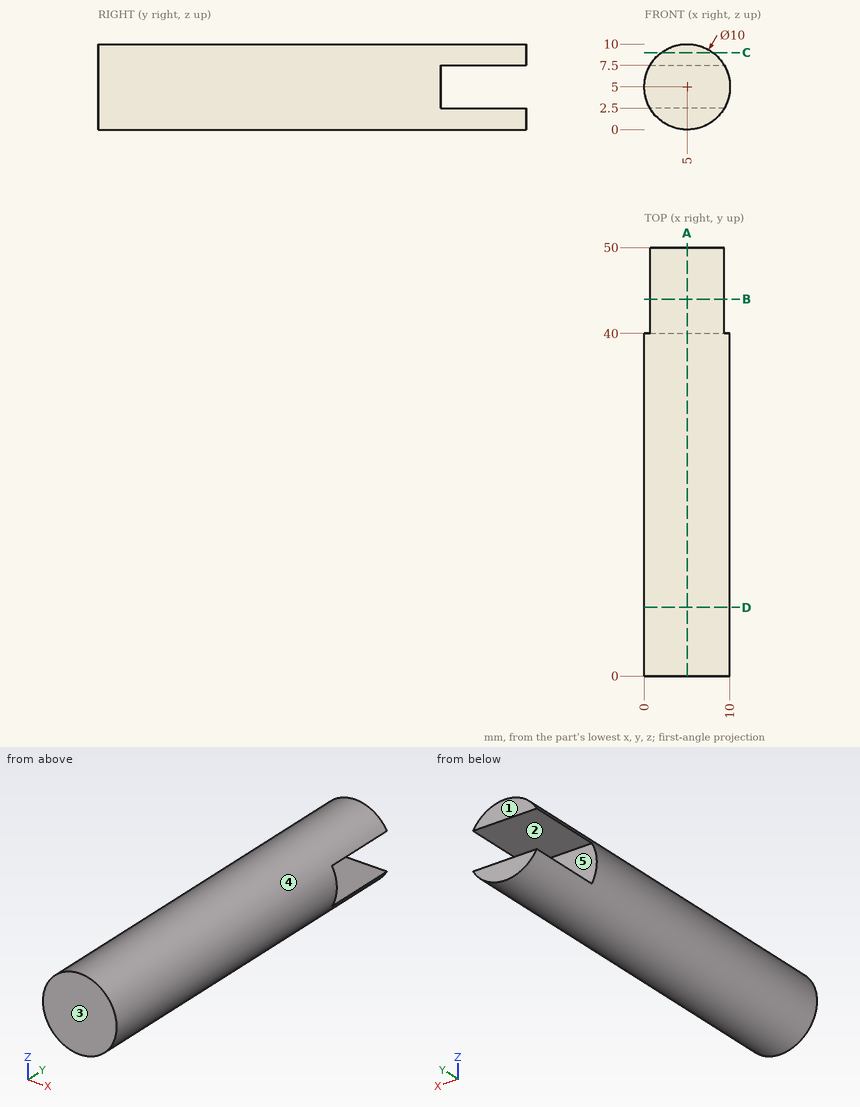
Source: three-view drawing plus pictorial views. Frame: mm from the lowest corner of the part. A direction names the side the tool comes from. Give positions to 0.01 mm unless a question says otherwise; leave off trailing zeros. Order: outer loops, then holes, each group sorted by start corner. A loop starts at its lowest first (then second) coordinate and runs counter-clockwise, first axis right, second up. Notation, with made-up numbers: M -34,-19 L -18,-19 A11 ccw -18,-4 Z; hole C 77.5,23.5 d5. An arc over 180 degrees is marked long. Return JSON: item names as keys, results as strings.
Item 1: First-contact query: P1, Ø1, axis at y = 38, z = 4, coming from the +X side; P2, Ø1.5, axis at x = 8, y = 44.5, coming from the -Z side; P3, Ø4, axis at x = 4, z = 4, coming from the +Y side; P4, Ø1, axis at y = 24, z = 8, coming from the -X side. Flat tips, straight axial feed; report the tip coordinate or a pass-through.
Solutions:
{"P1": "x = 9.97", "P2": "z = 0.53", "P3": "y = 50", "P4": "x = 0.67"}
Item 2: Cut plane C-C (z = 9). Return loops of the section in (x, y).
Solutions:
{"outline": "M 2,0 L 8,0 L 8,50 L 2,50 Z"}
Item 3: Cut plane B-B (y = 44). Return loops of the section in (x, z), then the cut area to 3 significant figures.
Solutions:
{"outline": "M 0.67,2.5 A5 ccw 9.33,2.5 Z; M 0.67,7.5 L 9.33,7.5 A5 ccw Z", "area": "30.7 mm^2"}
Item 4: Pull-direction query (Z, two-part tool) for the marked faces 3, 4 and 5; classes: +Z half, -Z half, draft (parallel to the pull), parting line (faces both ways), or undercut.
Solutions:
{"face 3": "draft", "face 4": "parting line", "face 5": "undercut"}
Item 5: Access query for the marked faces 1 and 2. Directions: +Z, -Z, +X, -X, +Y, -Y. A direction counts if a zero-diameter tool reaches every point of the face in a straight line with its end or side. Return the directions, or none.
Solutions:
{"face 1": "+Z, -Z, +X, -X, +Y", "face 2": "+X, -X, +Y"}
Item 6: Cut plane D-D (y = 8). Return loops of the section in (x, z), then the cut area to 3 significant figures.
Solutions:
{"outline": "C 5,5 d10", "area": "78.5 mm^2"}
Item 7: Cut plane A-A (x = 5). Return loops of the section in (y, z).
Solutions:
{"outline": "M 0,0 L 50,0 L 50,2.5 L 40,2.5 L 40,7.5 L 50,7.5 L 50,10 L 0,10 Z"}
Item 8: Ray query, probe 1 along Y at (x, z) = (4.5, 4.5); probe 2 along Z at (x, y) = (5.25, 19.5); probe 3 along X at (y, z) = (7, 2.5). Return the intervals inside material, ascending.
Solutions:
{"probe 1": "0 to 40", "probe 2": "0.01 to 9.99", "probe 3": "0.67 to 9.33"}
